Source: CAD feature listing. Evaluate the final solid. Frame: model axes, mm. Give positions to 0.01 mm unless a question says otherwise; leave off trailing zeros. Loops run counter-clockwise (first coordinate to the right, second up) from the corner with the lowest first, then second, coordinate; pieces in that order, holes last. Notation, with made-up numbers: M -11.75,30 L 27.25,30 A33 cw 27.25,65 Z; hole C 55.25,-2.75 d7. An arc over 180 degrees is marked long. Write item = value, one per line.
from build123d import *

# Parameters (mm, degrees)
SKETCH1_W               = 609.6
SKETCH1_H               = 304.8
BOSS_EXTRUDE1_DEPTH     = 3.175
SKETCH5_R               = 2.032
CUT_EXTRUDE4_DEPTH      = 4.175
SKETCH6_R               = 2.032
CUT_EXTRUDE5_DEPTH      = 10
CUT_EXTRUDE5_DEPTH_BACK = 3.175
SKETCH20_R              = 2.032
CUT_EXTRUDE17_DEPTH     = 4.175
SKETCH8_W               = 221.700000084
SKETCH8_H               = 139.7
CUT_EXTRUDE6_DEPTH      = 3.175
SKETCH19_W              = 14.489703264
SKETCH19_H              = 65.374013416
CUT_EXTRUDE16_DEPTH     = 4.175


with BuildPart() as part:
    # Sketch1 → Boss-Extrude1 (new body)
    with BuildSketch(Plane.XY):
        with Locations((-304.8, 152.4)):
            Rectangle(SKETCH1_W, SKETCH1_H)
    extrude(amount=BOSS_EXTRUDE1_DEPTH)

    # Sketch5 → Cut-Extrude4 (cut, through all)
    with BuildSketch(Plane.XY.offset(3.175)):
        with Locations((-533.4, 12.7)):
            Circle(SKETCH5_R)
        with Locations((-444.5, 12.7)):
            Circle(SKETCH5_R)
        with Locations((-355.6, 12.7)):
            Circle(SKETCH5_R)
        with Locations((-266.7, 12.7)):
            Circle(SKETCH5_R)
        with Locations((-177.8, 12.7)):
            Circle(SKETCH5_R)
        with Locations((-88.9, 12.7)):
            Circle(SKETCH5_R)
        with Locations((-88.9, 292.1)):
            Circle(SKETCH5_R)
        with Locations((-177.8, 292.1)):
            Circle(SKETCH5_R)
        with Locations((-266.7, 292.1)):
            Circle(SKETCH5_R)
        with Locations((-355.6, 292.1)):
            Circle(SKETCH5_R)
        with Locations((-444.5, 292.1)):
            Circle(SKETCH5_R)
        with Locations((-533.4, 292.1)):
            Circle(SKETCH5_R)
    extrude(amount=-CUT_EXTRUDE4_DEPTH, mode=Mode.SUBTRACT)

    # Sketch6 → Cut-Extrude5 (cut, two sides)
    with BuildSketch(Plane.XY.offset(3.175)) as cut_extrude5_sk:
        with Locations((-596.9, 254)):
            Circle(SKETCH6_R)
        with Locations((-596.9, 114.3)):
            Circle(SKETCH6_R)
        with Locations((-596.9, 44.45)):
            Circle(SKETCH6_R)
        with Locations((-12.7, 254)):
            Circle(SKETCH6_R)
        with Locations((-12.7, 184.15)):
            Circle(SKETCH6_R)
        with Locations((-12.7, 114.3)):
            Circle(SKETCH6_R)
        with Locations((-12.7, 44.45)):
            Circle(SKETCH6_R)
    extrude(amount=CUT_EXTRUDE5_DEPTH, mode=Mode.SUBTRACT)
    extrude(cut_extrude5_sk.sketch, amount=-CUT_EXTRUDE5_DEPTH_BACK, mode=Mode.SUBTRACT)

    # Sketch20 → Cut-Extrude17 (cut, through all)
    with BuildSketch(Plane.XY.offset(3.175)):
        with Locations((-597.110646497, 175.018670592)):
            Circle(SKETCH20_R)
        with Locations((-597.110646497, 206.768670592)):
            Circle(SKETCH20_R)
    extrude(amount=-CUT_EXTRUDE17_DEPTH, mode=Mode.SUBTRACT)

    # Sketch8 → Cut-Extrude6 (cut)
    with BuildSketch(Plane.XY.offset(3.175)):
        with Locations((-454.183579328, 196.85)):
            Rectangle(SKETCH8_W, SKETCH8_H)
    extrude(amount=-CUT_EXTRUDE6_DEPTH, mode=Mode.SUBTRACT)

    # Sketch19 → Cut-Extrude16 (cut, through all)
    with BuildSketch(Plane(origin=(0, 0, 0), x_dir=(-1, 0, 0), z_dir=(0, 0, -1))):
        with Locations((572.278431002, 192.206332301)):
            Rectangle(SKETCH19_W, SKETCH19_H)
    extrude(amount=-CUT_EXTRUDE16_DEPTH, mode=Mode.SUBTRACT)


solid = part.part
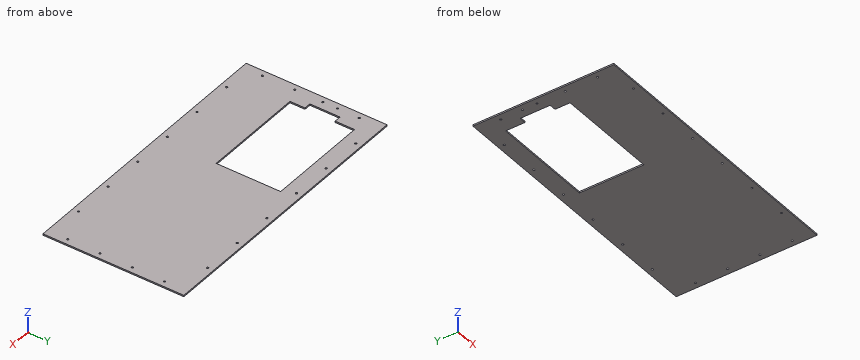
1. Cut plane A-A, the plane y = 138. Return the cut outline in (x, z) (3 decimals), then the cut area to 3 significant figures.
Derived:
outline = M -609.6,0 L -565.034,0 L -565.034,3.175 L -609.6,3.175 Z; M -343.334,0 L 0,0 L 0,3.175 L -343.334,3.175 Z
area = 1,230 mm²
2. Material intervals for probe 1 along X at (y, z) = (44.5, 2.65); probe 2 along Y at (x, z) = (-266.7, 1.95); probe 3 along Y at (x, z) = (-596.9, 2.5), sorted ascending. Write a range as from..to.
Derived:
probe_1 = -609.6..-598.93, -594.87..-14.73, -10.67..0
probe_2 = 0..10.67, 14.73..290.07, 294.13..304.8
probe_3 = 0..42.42, 46.48..112.27, 116.33..173, 177.04..204.75, 208.79..251.97, 256.03..304.8
3. Cut plane C-C, the plane z = 0.5. Count the separate pieces of the cut face and the enclosed holes in it, then the cut area to 3 significant figures.
Derived:
separate_pieces = 1
enclosed_holes = 22
area = 154,000 mm²
4. Cut plane B-B, the plane x = -379. Return the cut outline in (y, z) (3 decimals).
Derived:
outline = M 0,0 L 127,0 L 127,3.175 L 0,3.175 Z; M 266.7,0 L 304.8,0 L 304.8,3.175 L 266.7,3.175 Z
